For this review, use the dimensioned drawing (mm, ordinates from the lowest corner) and the shaded views. A direction names the side the tool comes from. Coordinates: 2 decimals unless noted, no trailing zeros. Order: outer loops, then holes, each group sorted by start corner. A loop starts at its lowest first (then second) coordinate and runs counter-clockwise, first axis right, second up. Notation, with made-up numbers: M 20.25,-10.75 L 63.25,-10.75 A27 ccw 63.25,26.25 Z; hole C 21,31.5 d6. An arc over 180 degrees is marked long. Answer in a Markdown table with one row per item.
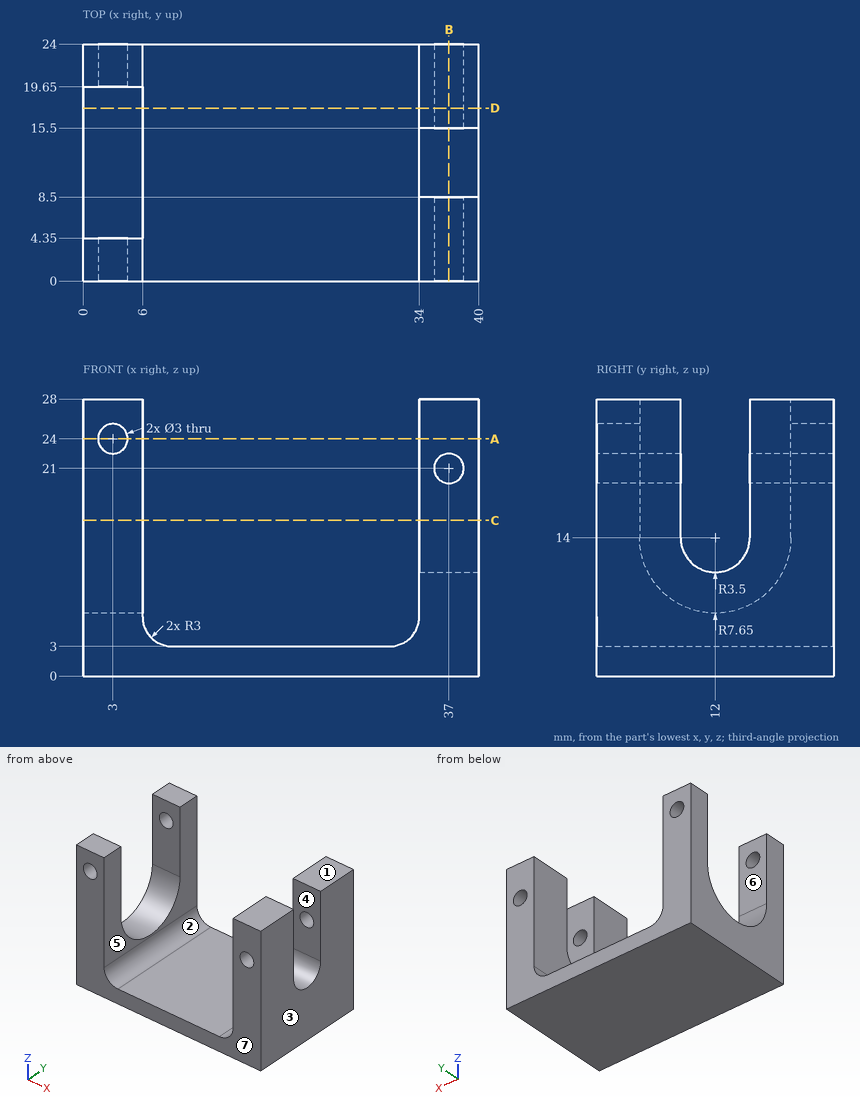
(1) Add section D-D, the plane y = 17.5. Give the boundary of the cut face in (x, z), and give its area (3 significant figures).
Return value:
| item | result |
|---|---|
| outline | M 0,0 L 40,0 L 40,28 L 34,28 L 34,6 A3 cw 31,3 L 9,3 A3 cw 6,6 L 6,8.68 L 0,8.68 Z; hole C 37,21 d3 |
| area | 301 mm2 |
(2) For line 1 along Z through (x, y) = (3, 23.15); line 2 along Z through (x, y) = (37, 2.25); line 3 along X through (y, z) = (2, 12), list the stretches that pass through material, from the lowest coordinate up. Write a range as from..to.
Return value:
| item | result |
|---|---|
| line 1 | z = 0..22.5, 25.5..28 |
| line 2 | z = 0..19.5, 22.5..28 |
| line 3 | x = 0..6, 34..40 |
(3) Add section B-B, the plane x = 37. Give the boundary of the cut face in (y, z).
Return value:
| item | result |
|---|---|
| outline | M 0,0 L 24,0 L 24,19.5 L 15.5,19.5 L 15.5,14 A3.5 cw 8.5,14 L 8.5,19.5 L 0,19.5 Z; M 0,22.5 L 8.5,22.5 L 8.5,28 L 0,28 Z; M 15.5,22.5 L 24,22.5 L 24,28 L 15.5,28 Z |
(4) Insertion check: pin 1 Ø4 at (x, z) = (3, 24) entering from -Y; pin 2 Ø5 at (y, z) = (12.5, 16) entering from -X (3 decimals); pin 3 Ø1 at (x, y) = (28.5, 8.5) entering from +Z. Each pin has a flat end and moves straight along its axis. Give the tip position at first contact, or say it passes through.
Return value:
| item | result |
|---|---|
| pin 1 | stops at y = 0 |
| pin 2 | passes through |
| pin 3 | stops at z = 3 |
(5) For the marked faces 4, 5, 6 and 7, list the 3-axis set-ups (+Z, -Z, +X, -X, +Y, -Y) from which the entire face can be reached by the end or side of a thin tool; tool diameter is ignored.
Return value:
| item | result |
|---|---|
| face 4 | +Z, +X, -X |
| face 5 | +Z, +Y, -Y |
| face 6 | +Z, -X |
| face 7 | +Z, -Z, +X, -X, -Y |
(6) Add section C-C, the plane z = 15.75. Give the boundary of the cut face in (x, y), and give its area (3 significant figures).
Return value:
| item | result |
|---|---|
| outline | M 0,0 L 6,0 L 6,4.35 L 0,4.35 Z; M 0,19.65 L 6,19.65 L 6,24 L 0,24 Z; M 34,0 L 40,0 L 40,8.5 L 34,8.5 Z; M 34,15.5 L 40,15.5 L 40,24 L 34,24 Z |
| area | 154 mm2 |
(7) Draft analysis for pull direction X (two halves, no side actions). For the marked faces 1, 2 and 3, state which applies: pulls with the +X half, pulls with the -X half, needs draft (parallel to the pull), parting line crosses it, or undercut.
Return value:
| item | result |
|---|---|
| face 1 | needs draft |
| face 2 | undercut |
| face 3 | pulls with the +X half |
(8) Add section A-A, the plane z = 24. Give the boundary of the cut face in (x, y), and give its area (3 significant figures).
Return value:
| item | result |
|---|---|
| outline | M 0,0 L 1.5,0 L 1.5,4.35 L 0,4.35 Z; M 0,19.65 L 1.5,19.65 L 1.5,24 L 0,24 Z; M 4.5,0 L 6,0 L 6,4.35 L 4.5,4.35 Z; M 4.5,19.65 L 6,19.65 L 6,24 L 4.5,24 Z; M 34,0 L 40,0 L 40,8.5 L 34,8.5 Z; M 34,15.5 L 40,15.5 L 40,24 L 34,24 Z |
| area | 128 mm2 |
